from build123d import *

# Parameters (mm, degrees)
BOSS_EXTRUDE1_DEPTH = 19.05


with BuildPart() as part:
    # Sketch3 → Boss-Extrude1 (new body)
    with BuildSketch(Plane(origin=(0, 0, 0), x_dir=(1, 0, 0), z_dir=(0, 1, 0))):
        with BuildLine():
            Line((-5.541525375, 3.58326618), (-2.47962532, 5.150959008))
            Line((-2.47962532, 5.150959008), (-2.47962532, 6.474170352))
            ThreePointArc((-2.47962532, 6.474170352), (-2.221563685, 14.417025562), (4.617359972, 10.369227654))
            ThreePointArc((4.617359972, 10.369227654), (4.047797908, 8.147663968), (2.47962532, 6.474170352))
            Line((2.47962532, 6.474170352), (2.47962532, 5.20231788))
            Line((2.47962532, 5.20231788), (5.873962228, 3.007468661))
            Line((5.873962228, 3.007468661), (5.541525375, -3.58326618))
            Line((5.541525375, -3.58326618), (4.701204968, -4.013510228))
            Line((4.701204968, -4.013510228), (4.701204968, -6.905610932))
            Line((4.701204968, -6.905610932), (5.918780254, -8.378526195))
            ThreePointArc((5.918780254, -8.378526195), (9.922634137, -0.265088751), (6.526624698, 8.120961152))
            ThreePointArc((6.526624698, 8.120961152), (5.706991897, 14.686716316), (0, 18.035026682))
            ThreePointArc((0, 18.035026682), (-5.706991897, 14.686716316), (-6.526624698, 8.120961152))
            ThreePointArc((-6.526624698, 8.120961152), (-9.922634137, -0.265088751), (-5.918780254, -8.378526195))
            Line((-5.918780254, -8.378526195), (-4.701204968, -6.905610932))
            Line((-4.701204968, -6.905610932), (-4.701204968, -3.765798027))
            Line((-4.701204968, -3.765798027), (-5.873962228, -3.007468661))
            Line((-5.873962228, -3.007468661), (-5.541525375, 3.58326618))
        make_face()
        with BuildLine():
            Line((-2.47962532, 6.474170352), (-2.47962532, 5.150959008))
            Line((-2.47962532, 5.150959008), (-1.063503338, 5.876013463))
            ThreePointArc((-1.063503338, 5.876013463), (-1.79663243, 6.115743784), (-2.47962532, 6.474170352))
        make_face()
        with BuildLine():
            ThreePointArc((2.47962532, 6.474170352), (1.921985685, 6.17089654), (1.328021538, 5.946968965))
            Line((1.328021538, 5.946968965), (2.47962532, 5.20231788))
            Line((2.47962532, 5.20231788), (2.47962532, 6.474170352))
        make_face()
    extrude(amount=BOSS_EXTRUDE1_DEPTH)

    # Fillet6
    # a fillet whose section is not a circle: 1.27 mm, written as the material it takes off along each edge
    with BuildSketch(Plane(origin=(1.328021538, -5.283304691, -5.946968965), x_dir=(0.8397378391322112, 0, 0.5429920455490709), z_dir=(0, 1, 0))) as fillet6_piece_1:
        with BuildLine():
            Bezier((2.113321876, 0), (0.3966534, 0), (0.898889741, 1.641556979), weights=[1, 0.118948346, 1])
            ThreePointArc((0.898889741, 1.641556979), (0.533488386, 0.774757636), (0, 0))
            Line((0, 0), (2.113321876, 0))
        make_face()
    extrude(amount=29.616609382, mode=Mode.SUBTRACT)
    with BuildSketch(Plane(origin=(-1.063503338, -6.120582224, -5.876013463), x_dir=(-0.891835980226881, 0, -0.4523589110128793), z_dir=(0, 1, 0))) as fillet6_piece_2:
        with BuildLine():
            Bezier((2.168149873, 0), (0.323600022, 0.445521101), (1.438773255, 1.980852292), weights=[1, 0.11123936, 1])
            Line((1.438773255, 1.980852292), (0, 0))
            ThreePointArc((0, 0), (1.084074937, 0.129064678), (2.168149873, 0))
        make_face()
    extrude(amount=31.291164449, mode=Mode.SUBTRACT)


solid = part.part
Geometry: final body of the model. Coordinates: model frame, mm. A direction names the side the tool comes from. Give positions to 0.01 mm unless a question says otherwise; leave off trailing zeros. Write each loop counter-clockwise with the first axis right and the second up, starting at its lowest first coordinate (ties: lowest second). Pieces come first, ordered by that corner, then holes. Notation, with made-up numbers: M 35,-3.75 L 82,-3.75 A28 ccw 82,22.25 Z; hole C 10,27.5 d9. An arc over 180 degrees is marked long. Answer in a Markdown table with one row per item. Add a question column.
(1) Section B-B on x = -7.25. Return loops of the section in (y, z).
(2) Ray query, line 1 (X direction, y = 10, z = -8.5); line 2 (X direction, y = 9, z = -14.5); line 3 (Z direction, x = 8.25, y = 16.5). Return the intervals inside material, ascending.
(3) First-contact query: pin 1 (3 mm diameter, centred on x = -2, y = 14.5, fed in from +Z); pin 2 (1.6 mm diameter, centred on y = 12, z = 6, fed in from +X); pin 3 (10 mm diameter, centred on y = 15, z = -4, fed in from -X); pin 4 (5 mm diameter, centred on y = 4, z = -8, fed in from -X). Flat tips, straight axial feed; report the tip coordinate or a pass-through.
(4) Section C-C on x = -1. Return loops of the section in (y, z).
(5) Reachability of faces 4 (the cylindrical face through (5.759, 9.392, -14.606)), 5 (the flat face through (-5.71, 9.39, -0.24)), 6 (the flat face through (5.3, 9.39, 7.63)) from +Z, -Z, +X, -X, +Y, -Y: full face, straight path, thin tool, end or side. Return the list, or none.
(6) Mould query, pull axis X, two halves, no side actions, for faces 1 (the flat face through (-5.28, 9.39, 3.39)), 2 (the cylindrical face through (-9.927, 9.392, 0.135)), 3 (the cylindrical face through (9.917, 9.392, 0.395)). Classes: +X half, -X half, draft (parallel to the pull), parting line (faces both ways), or undercut.
(7) Section A-A on x = 4. Return loops of the section in (y, z), and give its area (3 significant figures).
Result set:
| question | item | result |
|---|---|---|
| 1 | outline | M 0,-7.36 L 19.05,-7.36 L 19.05,7.07 L 0,7.07 Z |
| 2 | line 1 | x = -6.65 to -4.22, 4.22 to 6.65 |
| 2 | line 2 | x = -5.83 to -2.06, 2.06 to 5.83 |
| 2 | line 3 | z = -6 to 5.72 |
| 3 | pin 1 | stops at z = -4.63 |
| 3 | pin 2 | stops at x = 8.55 |
| 3 | pin 3 | stops at x = -9.93 |
| 3 | pin 4 | stops at x = -8.54 |
| 4 | outline | M 0,-17.89 L 19.05,-17.89 L 19.05,-14.88 L 0,-14.88 Z |
| 5 | face 4 | +X, +Y, -Y |
| 5 | face 5 | +Y, -Y |
| 5 | face 6 | +Z, +Y, -Y |
| 6 | face 1 | undercut |
| 6 | face 2 | -X half |
| 6 | face 3 | +X half |
| 7 | outline | M 0,-16.52 L 19.05,-16.52 L 19.05,-12.68 L 0,-12.68 Z; M 0,-8.06 L 19.05,-8.06 L 19.05,-4.22 L 0,-4.22 Z |
| 7 | area | 146 mm^2 |
